from build123d import *

# Parameters (mm, degrees)
ESQUISSE1_R             = 5
BASE_EXTRUSION_DEPTH    = 6
ESQUISSE2_R             = 3.201580403
BOSS_EXTRU_1_DEPTH      = 20
ENL_V_MAT_EXTRU_1_DEPTH = 5
CONG_1_R                = 0.5
CHANFREIN1_SIZE         = 1


with BuildPart() as part:
    # Esquisse1 → Base-Extrusion (new body)
    with BuildSketch(Plane.XY):
        Circle(ESQUISSE1_R)
    extrude(amount=BASE_EXTRUSION_DEPTH)

    # Esquisse2 → Boss.-Extru.1 (add)
    with BuildSketch(Plane(origin=(0, 0, 0), x_dir=(-1, 0, 0), z_dir=(0, 0, -1))):
        Circle(ESQUISSE2_R)
    extrude(amount=BOSS_EXTRU_1_DEPTH)

    # Esquisse3 → Enlèv. mat.-Extru.1 (cut)
    with BuildSketch(Plane.XY.offset(6)):
        Polygon((3.140063694, 0), (1.240063694, 2.5), (-1.240063694, 2.5), (-3.140063694, 0), (-1.240063694, -2.5), (1.240063694, -2.5), align=None)
    extrude(amount=-ENL_V_MAT_EXTRU_1_DEPTH, mode=Mode.SUBTRACT)

    # Congé1
    cong_1_edges = [part.edges().sort_by_distance(p)[0] for p in [
        (-5, 0, 6),
    ]]
    fillet(cong_1_edges, radius=CONG_1_R)

    # Chanfrein1
    chanfrein1_edges = [part.edges().sort_by_distance(p)[0] for p in [
        (3.201580403, 0, -20),
    ]]
    chamfer(chanfrein1_edges, length=CHANFREIN1_SIZE)


solid = part.part
Can you work these out from the model? Positions are in its coordinate system, mm. A direction names the side the tool comes from. Round coordinates to 2 decimals unless told otherwise and drop trailing zeros. Order: outer loops, then holes, each group sorted by start corner. A loop starts at its lowest first (then second) coordinate and runs counter-clockwise, first axis right, second up. Notation, with made-up numbers: (55, -19) - (98, -19) arc R26 ccw to (98, 16) - close; hole circle Ø8 at (52.25, 11.25). An arc over 180 degrees is marked (long way). Answer in a Markdown table with one row per item.
(1) Suppose I cut it at A-A, the plane x = 0. Please give me the cut outline in (y, z).
From the geometry:
| item | result |
|---|---|
| outline | (-5, 0) - (-3.2, 0) - (-3.2, -19) - (-2.2, -20) - (2.2, -20) - (3.2, -19) - (3.2, 0) - (5, 0) - (5, 5.5) arc R0.5 ccw to (4.5, 6) - (2.5, 6) - (2.5, 1) - (-2.5, 1) - (-2.5, 6) - (-4.5, 6) arc R0.5 ccw to (-5, 5.5) - close |
(2) Please list where these lines run through material, in increasing order: L1, parallel to Z at x = 4, y = 1.75; L2, parallel to Y at x = 1.5, z = 3.25; L3, parallel to Y at x = 0, z = -17.75. Write a range as from..to.
From the geometry:
| item | result |
|---|---|
| L1 | z = 0..6 |
| L2 | y = -4.77..-2.16, 2.16..4.77 |
| L3 | y = -3.2..3.2 |
(3) If we mould it in two halves opening along Y, with no side actions, what happens to faces 1 (the face through (2, -2, 6)), 2 (the face through (-3.054, 0.962, -9.367)), 3 (the face through (2.203, 1.233, 3.535))? For each: released by +Y, released by -Y, zero draft, split by the parting line, or undercut.
From the geometry:
| item | result |
|---|---|
| face 1 | zero draft |
| face 2 | split by the parting line |
| face 3 | undercut |
(4) For P1, Ø1.5, axis at x = -0.5, y = 0, coming from the +Z side; P2, Ø3, axis at x = -1.5, z = -4.5, coming from the +Y side; P3, Ø4, axis at x = 2.5, y = -4, coming from the -Z side, each with a flat end and sliding along its axis, tell me the tip position at first contact or that it passes through.
From the geometry:
| item | result |
|---|---|
| P1 | stops at z = 1 |
| P2 | stops at y = 3.2 |
| P3 | stops at z = -19.48 |
(5) Which directions (+Z, -Z, +X, -X, +Y, -Y) give clear straight access to the entire face, cutting with the end or side of a thin tool? Please do faces 4 (the face through (1, -3.3, 0)), 5 (the face through (-2.203, -1.233, 3.535)), 6 (the face through (0, 0, -20)).
From the geometry:
| item | result |
|---|---|
| face 4 | -Z |
| face 5 | +Z |
| face 6 | -Z, +X, -X, +Y, -Y |
(6) Suppose I cut it at B-B, the plane z = -6.75. Please give me the cut outline in (x, y).
From the geometry:
| item | result |
|---|---|
| outline | circle Ø6.4 at (0, 0) |
